Could you check a few things on this model? Use its own coordinates, in mm. Give positions to 0.01 mm unless a question says otherwise; leave off trailing zeros. Answer as CSV lines item,"result". Start each with the question number.
Q1. If I drill on line 1 along Z through (x, y) = (208, 5); line 2 along Y through (x, z) = (257.5, -1.5); line 3 along Z through (x, y) = (120, -15), over which ranges is the centre line in solid material (lowest first)?
Q2. Will these pins go through, and if not, where does the flat tip stop? pin 1 Ø0.8 at (x, z) = (339, 17.5) entering from -Y; pin 2 Ø1.9 at (x, z) = (138.5, 1) entering from -Y; pin 3 Ø3 at (x, y) = (374.5, -18.5) entering from +Z.
Q3. Imagine slicing it at A-A on x = 322. State how many separate pieces and enclosed holes the cut face has, and give its area (3 significant figures).
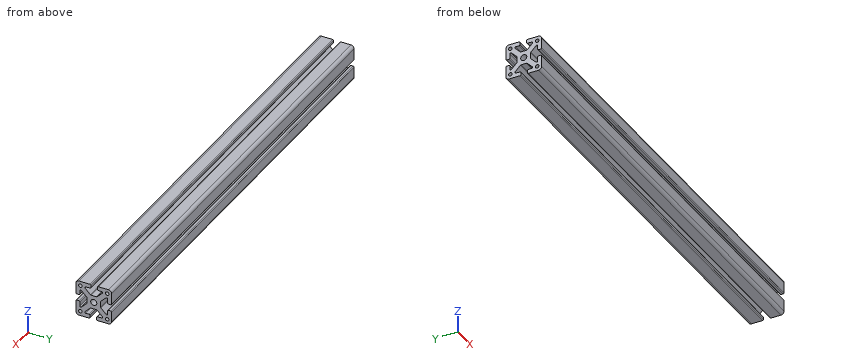
Autodesk Fusion 360 part; units mm, degrees
sketch "Sketch1" plane through (0, 0, 0) normal (1, 0, 0) x (0, 1, 0)
  line L0 (0, 0) -> (0, 40) construction
  line L1 (0, 0) -> (40, 0) construction
  line L2 (0, 7.6) -> (3.1, 7.6)
  arc A0 (3.1, 7.6) -> (3.8071, 7.8929) centre (3.1, 8.6) ccw
  line L3 (3.8071, 7.8929) -> (9.7071, 13.7929)
  arc A1 (9.7071, 13.7929) -> (9, 15.5) centre (9, 14.5) ccw
  line L4 (9, 15.5) -> (5.1, 15.5)
  arc A2 (4.1, 16.5) -> (5.1, 15.5) centre (5.1, 16.5) ccw
  line L5 (4.1, 16.5) -> (4.1, 19)
  arc A3 (5.1, 20) -> (4.1, 19) centre (5.1, 19) ccw
  line L6 (5.1, 20) -> (16.5, 20)
  arc A4 (20, 16.5) -> (16.5, 20) centre (16.5, 16.5) ccw
  line L7 (20, 16.5) -> (20, 4.1)
  arc A5 (19, 3.1) -> (20, 4.1) centre (19, 4.1) ccw
  line L8 (19, 3.1) -> (16.5, 3.1)
  arc A6 (15.5, 4.1) -> (16.5, 3.1) centre (16.5, 4.1) ccw
  line L9 (15.5, 4.1) -> (15.5, 9)
  line L10 (7.6, 0) -> (7.6, 3.1)
  arc A7 (15.5, 9) -> (13.7929, 9.7071) centre (14.5, 9) ccw
  line L11 (13.7929, 9.7071) -> (7.8929, 3.8071)
  arc A8 (7.8929, 3.8071) -> (7.6, 3.1) centre (8.6, 3.1) ccw
  arc A9 (3.4, 0) -> (0, 3.4) centre (0, 0) ccw
  line L12 (0, 0) -> (3.4, 0) construction
  line L13 (0, 0) -> (0, 3.4) construction
  line L14 (0, 7.6) -> (0, 3.4)
  line L15 (3.4, 0) -> (7.6, 0)
  line L16 (-7.6, 0) -> (-3.4, 0)
  arc A10 (-3.8071, 7.8929) -> (-3.1, 7.6) centre (-3.1, 8.6) ccw
  line L17 (-7.6, 0) -> (-7.6, 3.1)
  arc A11 (-7.6, 3.1) -> (-7.8929, 3.8071) centre (-8.6, 3.1) ccw
  line L18 (0, 7.6) -> (-3.1, 7.6)
  line L19 (0, 3.4) -> (0, 7.6)
  arc A12 (0, 3.4) -> (-3.4, 0) centre (0, 0) ccw
  arc A13 (-13.7929, 9.7071) -> (-15.5, 9) centre (-14.5, 9) ccw
  line L20 (-20, 5.1) -> (-20, 16.5)
  arc A14 (-16.5, 20) -> (-20, 16.5) centre (-16.5, 16.5) ccw
  arc A15 (-20, 5.1) -> (-19, 4.1) centre (-19, 5.1) ccw
  arc A16 (-16.5, 4.1) -> (-15.5, 5.1) centre (-16.5, 5.1) ccw
  arc A17 (-9, 15.5) -> (-9.7071, 13.7929) centre (-9, 14.5) ccw
  line L21 (-7.8929, 3.8071) -> (-13.7929, 9.7071)
  line L22 (-15.5, 9) -> (-15.5, 5.1)
  line L23 (-16.5, 4.1) -> (-19, 4.1)
  arc A18 (-3.1, 19) -> (-4.1, 20) centre (-4.1, 19) ccw
  line L24 (-16.5, 20) -> (-4.1, 20)
  line L25 (-4.1, 15.5) -> (-9, 15.5)
  line L26 (-3.1, 19) -> (-3.1, 16.5)
  arc A19 (-4.1, 15.5) -> (-3.1, 16.5) centre (-4.1, 16.5) ccw
  line L27 (-9.7071, 13.7929) -> (-3.8071, 7.8929)
  line L28 (0, -7.6) -> (0, -3.4)
  arc A20 (-7.8929, -3.8071) -> (-7.6, -3.1) centre (-8.6, -3.1) ccw
  line L29 (0, -7.6) -> (-3.1, -7.6)
  arc A21 (-3.1, -7.6) -> (-3.8071, -7.8929) centre (-3.1, -8.6) ccw
  line L30 (-7.6, 0) -> (-7.6, -3.1)
  line L31 (-3.4, 0) -> (-7.6, 0)
  arc A22 (-3.4, 0) -> (0, -3.4) centre (0, 0) ccw
  arc A23 (-9.7071, -13.7929) -> (-9, -15.5) centre (-9, -14.5) ccw
  line L32 (-5.1, -20) -> (-16.5, -20)
  arc A24 (-20, -16.5) -> (-16.5, -20) centre (-16.5, -16.5) ccw
  arc A25 (-5.1, -20) -> (-4.1, -19) centre (-5.1, -19) ccw
  arc A26 (-4.1, -16.5) -> (-5.1, -15.5) centre (-5.1, -16.5) ccw
  arc A27 (-15.5, -9) -> (-13.7929, -9.7071) centre (-14.5, -9) ccw
  line L33 (-3.8071, -7.8929) -> (-9.7071, -13.7929)
  line L34 (-9, -15.5) -> (-5.1, -15.5)
  line L35 (-4.1, -16.5) -> (-4.1, -19)
  arc A28 (-19, -3.1) -> (-20, -4.1) centre (-19, -4.1) ccw
  line L36 (-20, -16.5) -> (-20, -4.1)
  line L37 (-15.5, -4.1) -> (-15.5, -9)
  line L38 (-19, -3.1) -> (-16.5, -3.1)
  arc A29 (-15.5, -4.1) -> (-16.5, -3.1) centre (-16.5, -4.1) ccw
  line L39 (-13.7929, -9.7071) -> (-7.8929, -3.8071)
  line L40 (7.6, 0) -> (3.4, 0)
  arc A30 (3.8071, -7.8929) -> (3.1, -7.6) centre (3.1, -8.6) ccw
  line L41 (7.6, 0) -> (7.6, -3.1)
  arc A31 (7.6, -3.1) -> (7.8929, -3.8071) centre (8.6, -3.1) ccw
  line L42 (0, -7.6) -> (3.1, -7.6)
  line L43 (0, -3.4) -> (0, -7.6)
  arc A32 (0, -3.4) -> (3.4, 0) centre (0, 0) ccw
  arc A33 (13.7929, -9.7071) -> (15.5, -9) centre (14.5, -9) ccw
  line L44 (20, -5.1) -> (20, -16.5)
  arc A34 (16.5, -20) -> (20, -16.5) centre (16.5, -16.5) ccw
  arc A35 (20, -5.1) -> (19, -4.1) centre (19, -5.1) ccw
  arc A36 (16.5, -4.1) -> (15.5, -5.1) centre (16.5, -5.1) ccw
  arc A37 (9, -15.5) -> (9.7071, -13.7929) centre (9, -14.5) ccw
  line L45 (7.8929, -3.8071) -> (13.7929, -9.7071)
  line L46 (15.5, -9) -> (15.5, -5.1)
  line L47 (16.5, -4.1) -> (19, -4.1)
  arc A38 (3.1, -19) -> (4.1, -20) centre (4.1, -19) ccw
  line L48 (16.5, -20) -> (4.1, -20)
  line L49 (4.1, -15.5) -> (9, -15.5)
  line L50 (3.1, -19) -> (3.1, -16.5)
  arc A39 (4.1, -15.5) -> (3.1, -16.5) centre (4.1, -16.5) ccw
  line L51 (9.7071, -13.7929) -> (3.8071, -7.8929)
  circle A40 centre (15, 15) radius 2
  circle A41 centre (-15, 15) radius 2
  circle A42 centre (-15, -15) radius 2
  circle A43 centre (15, -15) radius 2
  dimension "d26" = 40
  dimension "d27" = 40
  dimension "d31" = 20
  dimension "d32" = 3.5
  dimension "d33" = 7.6
  dimension "d35" = 4.5
  dimension "d36" = 1
  dimension "d37" = 1
  dimension "d38" = 1
  dimension "d39" = 1
  dimension "d40" = 4.5
  dimension "d41" = 4.1
  dimension "d42" = 4.1
  dimension "d43" = 16.5
  dimension "d44" = 7.6
  dimension "d45" = 1
  dimension "d46" = 1
  dimension "d47" = 1
  dimension "d48" = 1
  dimension "d49" = 9
  dimension "d50" = 9
  dimension "d51" = 1
  dimension "d52" = 1
  dimension "d53" = 3.4
  dimension "d54" = 90
  dimension "d56" = 360
  dimension "d60" = 4
  dimension "d61" = 15
  dimension "d62" = 15
extrude "Extrude2" add sketch "Sketch1" along normal blind 500 contours L2 A0 L3 A1 L4 A2 L5 A3 L6 A4 L7 A5 L8 A6 L9 L10 A7 L11 A8 A9 L14 L15 L19 L40 | L14 L16 A10 L17 A11 L18 L19 A12 A13 L20 A14 A15 A16 A17 L21 L22 L23 A18 L24 L25 L26 A19 L27 L31 | L15 L28 L40 A30 L41 A31 L42 L43 A32 A33 L44 A34 A35 A36 A37 L45 L46 L47 A38 L48 L49 L50 A39 L51 | L16 L28 A20 L29 A21 L30 L31 A22 A23 L32 A24 A25 A26 A27 L33 L34 L35 A28 L36 L37 L38 A29 L39 L43
equation "Length = 500 mm"
equation "d63 = Length"
Conclusion:
1,line 1,"-20 to -15.5, -9.09 to 9.09, 15.51 to 19.99"
1,line 2,"-7.6 to -3.05, 3.05 to 7.6"
1,line 3,"-20 to -17, -13 to -9.87, 9.87 to 13, 17 to 20"
2,pin 1,"y = -19.95"
2,pin 2,"y = -7.6"
2,pin 3,"z = 19.96"
3,separate pieces,"1"
3,enclosed holes,"5"
3,area,"908 mm^2"
